from build123d import *

# Parameters (mm, degrees)
SKETCH1_R           = 3
BOSS_EXTRUDE1_DEPTH = 20
CUT_EXTRUDE1_DEPTH  = 1.2


with BuildPart() as part:
    # Sketch1 → Boss-Extrude1 (new body)
    with BuildSketch(Plane(origin=(0, 0, 0), x_dir=(1, 0, 0), z_dir=(0, 1, 0))):
        with Locations(Location((0, 0, 0), (0, 0, 270))):
            Circle(SKETCH1_R)
    extrude(amount=BOSS_EXTRUDE1_DEPTH)

    # Sketch2 → Revolve1 (revolve)
    with BuildSketch(Plane.XY):
        with BuildLine():
            Line((0, 0), (0, -5))
            Line((0, -5), (-5.5, -5))
            ThreePointArc((-5.5, -5), (-6.207106781, -4.707106781), (-6.5, -4))
            Line((-6.5, -4), (-6.5, -1))
            ThreePointArc((-6.5, -1), (-6.207106781, -0.292893219), (-5.5, 0))
            Line((-5.5, 0), (0, 0))
        make_face()
    revolve(axis=Axis((0, 0, 0), (0, -1, 0)))

    # Sketch3 → Cut-Extrude1 (cut)
    with BuildSketch(Plane.XZ.offset(5)):
        Polygon((0.6, 8.375375313), (-0.6, 8.375375313), (-0.6, 0.8), (-0.8, 0.6), (-7.394108803, 0.6), (-7.394108803, -0.6), (-0.8, -0.6), (-0.6, -0.8), (-0.6, -7.930485814), (0.6, -7.930485814), (0.6, -0.8), (0.8, -0.6), (8.840235389, -0.6), (8.840235389, 0.6), (0.8, 0.6), (0.6, 0.8), align=None)
    extrude(amount=-CUT_EXTRUDE1_DEPTH, mode=Mode.SUBTRACT)


solid = part.part
Can you work these out from the model? Positions are in its coordinate system, mm. A direction names the side the tool comes from. Round coordinates to 2 decimals unless told otherwise and drop trailing zeros. Write each loop counter-clockwise with the first axis right and the second up, starting at its lowest first coordinate (ties: lowest second). Pieces come first, ordered by that corner, then holes. Notation, with made-up numbers: M 69.5,-15 L 74.5,-15 A31 ccw 74.5,16 Z; hole C -19.5,83.25 d5. An arc over 180 degrees is marked long. Use a Markdown table: item, result.
Item 1: I want a section at D-D (y = 9.75). List the corners of the cut face in (x, z) for me.
Found:
| item | result |
|---|---|
| outline | C 0,0 d6 |
Item 2: If I drill on line 1 along Y through (x, z) = (-1.75, -4.25); line 2 along Y through (x, z) = (-0.5, -0.25); line 3 along X through (y, z) = (-2.5, -2.25), over which ranges is the centre line in solid material (lowest first)? Write a range as [from, to].
Found:
| item | result |
|---|---|
| line 1 | y = [-5, 0] |
| line 2 | y = [-3.8, 20] |
| line 3 | x = [-6.1, 6.1] |
Item 3: I want a section at B-B (z = 0). List the corners of the cut face in (x, y) for me, and give its area (3 significant figures).
Found:
| item | result |
|---|---|
| outline | M -6.5,-3.8 L 6.5,-3.8 L 6.5,-1 A1 ccw 5.5,0 L 3,0 L 3,20 L -3,20 L -3,0 L -5.5,0 A1 ccw -6.5,-1 Z |
| area | 169 mm2 |
Item 4: We'd pull the mould along X, two halves only. Please class faces 1 (the face through (-6.2, -2.48, -1.95)), 2 (the face through (4, -4, 0.6)), 3 (the face through (-0.6, -4, -4)): released by +X, released by -X, zero draft, split by the parting line, or undercut.
Found:
| item | result |
|---|---|
| face 1 | split by the parting line |
| face 2 | zero draft |
| face 3 | undercut |
Item 5: Which directions (+Z, -Z, +X, -X, +Y, -Y) give clear straight access to the entire face, cutting with the end or side of a thin tool? Please do faces 4 (the face through (-4, -4, -0.6)), 5 (the face through (0.6, -4, -4)), 6 (the face through (0, -3.8, 0)), 7 (the face through (-2.4, 0, 2.4)), 8 (the face through (2, -5, 2)).
Found:
| item | result |
|---|---|
| face 4 | +X, -X, -Y |
| face 5 | +Z, -Z, -Y |
| face 6 | -Y |
| face 7 | +Y |
| face 8 | +Z, -Z, +X, -X, -Y |
Item 6: For pin 1 Ø2 at (x, y) = (2.5, 6) entering from -Z; pin 2 Ø0.6 at (y, z) = (-4.5, -3) entering from +X; pin 3 Ø5 at (x, y) = (4, 2) entering from +Z, each with a flat end and sliding along its axis, tell me the tip position at first contact or that it passes through.
Found:
| item | result |
|---|---|
| pin 1 | stops at z = -2.6 |
| pin 2 | stops at x = 5.83 |
| pin 3 | stops at z = 5.43 |
Item 7: I want a section at C-C (y = -1.5). List the corners of the cut face in (x, z) for me.
Found:
| item | result |
|---|---|
| outline | C 0,0 d13 |
Item 8: I want a section at A-A (x = 0). List the corners of the cut face in (y, z) for me, and give its area (3 significant figures).
Found:
| item | result |
|---|---|
| outline | M -3.8,-6.5 L -1,-6.5 A1 ccw 0,-5.5 L 0,-3 L 20,-3 L 20,3 L 0,3 L 0,5.5 A1 ccw -1,6.5 L -3.8,6.5 Z |
| area | 169 mm2 |
